Verification items for the finished model (mm, model axes). Round coordinates to 2 decimals unless told otherwise and drop trailing zeros. Loops run counter-clockwise (first coordinate to the right, second up) from the corner with the lowest first, then second, coordinate; pieces in that order, holes last. Notation, with made-up numbers: (-17, 1.25) -> (11, 1.25) arc R16 cw to (11, 25.25) -> close; hole circle Ø3 at (-21, 49). An arc over 180 degrees is marked (long way). Write item = value, one per line.
```python
from build123d import *

# Parameters (mm, degrees)
F0_R     = 20.6375
F0_R_2   = 33.3375
F1_DEPTH = 12.7


with BuildPart() as f1:
    # F0 (on Front) → F1 (new body)
    with BuildSketch(Plane.XZ):
        with BuildLine():
            Line((127, -87.2998), (62.387785, 51.261542))
            ThreePointArc((62.387785, 51.261542), (-55.078025, 82.736411), (-65.676996, -38.410384))
            Line((-65.676996, -38.410384), (214.566733, -318.654112))
            Line((214.566733, -318.654112), (386.016733, -318.654112))
            Line((386.016733, -318.654112), (375.971888, -255.233459))
            Line((375.971888, -255.233459), (127, -87.2998))
        make_face()
        with Locations((170.116733, -159.909192)):
            Circle(F0_R, mode=Mode.SUBTRACT)
        Circle(F0_R_2, mode=Mode.SUBTRACT)
    extrude(amount=F1_DEPTH)


solid = f1.part
```
(1) Sectioned sample at C-C, the plane z = 0. Record the cut outline in (x, y), and give its area (3 significant figures).
Filled sheet:
outline = (-86.92, -12.7) -> (-33.34, -12.7) -> (-33.34, 0) -> (-86.92, 0) -> close; (33.34, -12.7) -> (86.29, -12.7) -> (86.29, 0) -> (33.34, 0) -> close
area = 1,350 mm2
(2) Material ranges on probe 1 along X at (y, z) = (-1.5, -149.5); probe 2 along Z at (x, y) = (-6.5, -10.25); probe 3 along Z at (x, y) = (162.5, -1.5), recorded low to high. Write a range as from..to.
Filled sheet:
probe_1 = 45.41..152.3, 187.94..219.22
probe_2 = -97.59..-32.7, 32.7..97.03
probe_3 = -266.59..-179.09, -140.73..-111.24
(3) Sectioned sample at D-D, the plane z = -116.5. Record the cut outline in (x, y).
Filled sheet:
outline = (12.41, -12.7) -> (170.29, -12.7) -> (170.29, 0) -> (12.41, 0) -> close
(4) Sectioned sample at B-B, the plane x = 178. Record the cut outline in (y, z), and give its area (3 significant figures).
Filled sheet:
outline = (-12.7, -282.09) -> (0, -282.09) -> (0, -178.98) -> (-12.7, -178.98) -> close; (-12.7, -140.84) -> (0, -140.84) -> (0, -121.7) -> (-12.7, -121.7) -> close
area = 1,550 mm2
(5) Draft check along X on faces 1 (the face through (130, -12.7, -141)), 2 (the face through (153.74, -6.26, -172.47)), 3 (the face through (-53.476, -6.261, 83.829)). Enter one of: released by +X, released by -X, zero draft, split by the parting line, or undercut.
Filled sheet:
face_1 = zero draft
face_2 = undercut
face_3 = split by the parting line
(6) Go/stop test with flat-tipped pins: pin 1 Ø6 at (x, y) = (188, -11) entering from -Z; pin 2 Ø4 at (x, y) = (283.5, -3.5) entering from +Z; pin 3 Ø1 at (y, z) = (-9.5, -177.5) entering from -X. Record where each tip stops, or that it passes through.
Filled sheet:
pin_1 = -295.09
pin_2 = -191.51
pin_3 = 72.91
(7) Sectioned sample at A-A, the plane y = -3.75. Count the separate pieces of the cut face and the enclosed holes in it, and give its area (3 significant figures).
Filled sheet:
separate_pieces = 1
enclosed_holes = 2
area = 66,000 mm2
